CAD build for the part. Positions are in the model's coordinates, mm. Face numbers are marked on the shaded views. A direction names the side the tool comes from. Coordinates: 2 decimals unless noted, no trailing zeros. Loops run counter-clockwise (first coordinate to the right, second up) from the corner with the lowest first, then second, coordinate; pieces in that order, holes last. Notation, with made-up numbers: (88.5, 39.5) -> (108.5, 39.5) arc R12 cw to (108.5, 61.5) -> close; hole circle Ø2 at (17.5, 29). An arc over 180 degrees is marked (long way). Write item = value, one per line. Start each with the question number.
(1) Band-saw the part on A-A (z = 16.5). Write the cut outline in (x, y), and give its area (3 significant figures).
(2) Tool access for the marked faces 4, 5 and 6: list every direction of +Z, -Z, +X, -X, +Y, -Y with a clear straight run to the whole face (end or side of a thin tool).
(3) Band-saw the part on D-D (z = 7). Write the cut outline in (x, y).
(4) Band-saw the part on B-B (y = -22.5). Write the cut outline in (x, z), and give its area (3 significant figures).
(5) Drill centre lines: line 1 (Z direction, x = -35, y = -23); line 2 (X direction, y = -4.75, z = -4.5); line 3 (Z direction, x = 48, y = -4). Where is each one in solid material? Low to high. Write a range as from..to.
(6) Pull direction X, two halves, no side cores. Call the marked faces 1, 2 and 3: +X half, -X half, draft (parallel to the pull), parting line (faces both ways), or undercut.
(7) Band-saw the part on C-C (x = 48). Write the cut outline in (y, z).
(8) Flat gauge pins, fed straight in: P1, Ø4, axis at y = -5, z = -4, coming from the -X side; P2, Ø8, axis at x = 36.5, y = -10.5, coming from the +Z side; P3, Ø12.5, axis at x = 45, y = -12, coming from the +Z side. Where does each tip first touch, or does it go through?
```python
from build123d import *

# Parameters (mm, degrees)
F1_DEPTH = 25


with BuildPart() as f1:
    # F0 (on Front) → F1 (new body)
    with BuildSketch(Plane.XZ):
        with BuildLine():
            Line((-28.636673, -16.548831), (-62.88556, -16.548831))
            Line((-62.88556, -16.548831), (-62.88556, -22.880558))
            Line((-62.88556, -22.880558), (64.612396, -22.880558))
            Line((64.612396, -22.880558), (64.612396, -16.261026))
            Line((64.612396, -16.261026), (36.695234, -16.261026))
            Line((36.695234, -16.261026), (36.695234, 22.304947))
            Line((36.695234, 22.304947), (30.363506, 22.304947))
            ThreePointArc((30.363506, 22.304947), (3.355691, 4.127085), (-23.456169, 22.592753))
            Line((-23.456169, 22.592753), (-28.636673, 22.592753))
            Line((-28.636673, 22.592753), (-28.636673, -16.548831))
        make_face()
    extrude(amount=F1_DEPTH)


solid = f1.part
```
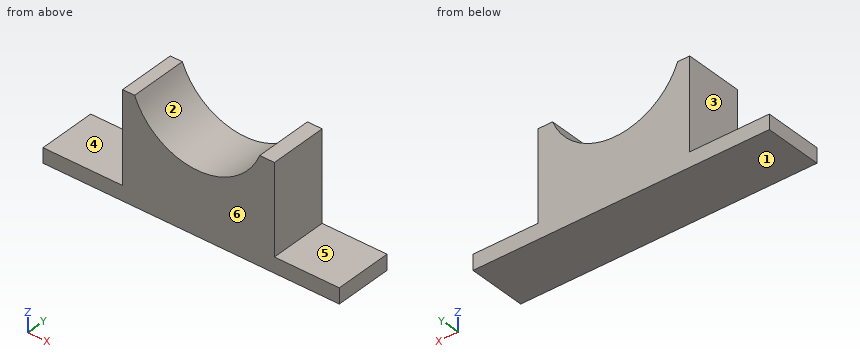
Findings below:
q1.outline = (-28.64, -25) -> (-20.21, -25) -> (-20.21, 0) -> (-28.64, 0) -> close; (27.23, -25) -> (36.7, -25) -> (36.7, 0) -> (27.23, 0) -> close
q1.area = 447 mm²
q2.face_4 = +Z, -X, +Y, -Y
q2.face_5 = +Z, +X, +Y, -Y
q2.face_6 = +Z, -Z, +X, -X, -Y
q3.outline = (-28.64, -25) -> (-9.06, -25) -> (-9.06, 0) -> (-28.64, 0) -> close; (16.08, -25) -> (36.7, -25) -> (36.7, 0) -> (16.08, 0) -> close
q4.outline = (-62.89, -22.88) -> (64.61, -22.88) -> (64.61, -16.26) -> (36.7, -16.26) -> (36.7, 22.3) -> (30.36, 22.3) arc R28.92 cw to (-23.46, 22.59) -> (-28.64, 22.59) -> (-28.64, -16.55) -> (-62.89, -16.55) -> close
q4.area = 2,650 mm²
q5.line_1 = -22.88..-16.55
q5.line_2 = -28.64..36.7
q5.line_3 = -22.88..-16.26
q6.face_1 = draft
q6.face_2 = undercut
q6.face_3 = -X half
q7.outline = (-25, -22.88) -> (0, -22.88) -> (0, -16.26) -> (-25, -16.26) -> close
q8.P1 = -28.64
q8.P2 = 22.3
q8.P3 = -16.26
